Verification items for the finished model (mm, model axes). A direction names the side the tool comes from. Coordinates: 2 decimals unless noted, no trailing zeros. Write each loop counter-clockwise with the first axis right and the second up, starting at its lowest first coordinate (ties: lowest second). Pieces come first, ordered by that corner, then holes. Notation, with made-up numbers: (65, 59) -> (74, 59) arc R27 ccw to (74, 81) -> close; hole circle Ø7 at (27, -14). An arc over 180 degrees is marked (long way). Write item = value, one per line. Start each with the question number.
(1) Material ranges on probe 1 along X at (y, z) = (41, 1.5); probe 2 along Z at (x, y) = (8.4, 0), recorded low to high. Write a range as [from, to].
(2) Section check B-B (y = 0). Record the cut outline in (x, z).
(3) Set-up check for faces 1 (the face through (-8, -0.7, -5.4)), 2 (the face through (0, -1, -9.5)): record each of +Z, -Z, +X, -X, +Y, -Y from which the full face is reachable in a straight line by a thin tool's end or side.
(4) Section check C-C (x = -1.75). Record the cut outline in (y, z).
(5) Section check D-D (z = -3). Record the cut outline in (x, y), plus the area to 3 significant figures.
(6) Mould release check, pull along X, two halves, no side actions. Record for faces 3 (the face through (8, -0.7, -5.4)), 4 (the face through (9.5, -1, -6)), 5 (the face through (8.76, -1.08, -4.88)): released by +X, released by -X, zero draft, split by the parting line, or undercut.
(7) Gauge pin test, flat end, axial feed: pin 1 Ø3 at (x, z) = (3, -6) entering from -Y. Record the tip position at first contact, or that the pin passes through.
(8) Section check A-A (z = 6.5). Record the cut outline in (x, y), plus the area to 3 significant figures.
```python
from build123d import *

# Parameters (mm, degrees)
F0_W     = 19
F0_H     = 19
F0_W_2   = 16
F0_H_2   = 16
F2_DEPTH = 50
F1_R     = 5
F3_DEPTH = 12.5
F4_R     = 1


with BuildPart() as f2:
    # F0 (on Front) → F2 (new body, symmetric)
    with BuildSketch(Plane.XZ):
        Rectangle(F0_W, F0_H)
        Rectangle(F0_W_2, F0_H_2, mode=Mode.SUBTRACT)
    extrude(amount=F2_DEPTH, both=True)

    # F1 (on Right) → F3 (cut, symmetric)
    with BuildSketch(Plane.YZ):
        Circle(F1_R)
    extrude(amount=F3_DEPTH, both=True, mode=Mode.SUBTRACT)

    # F4
    f4_edges = [f2.edges().sort_by_distance(p)[0] for p in [
        (9.5, 0, 9.5),
        (-9.5, 0, 9.5),
        (9.5, 0, -9.5),
        (-9.5, 0, -9.5),
    ]]
    fillet(f4_edges, radius=F4_R)


solid = f2.part
```
Response:
q1.probe_1 = [-9.5, -8], [8, 9.5]
q1.probe_2 = [-9.5, -5], [5, 9.5]
q2.outline = (-9.5, -8.5) arc R1 ccw to (-8.5, -9.5) -> (8.5, -9.5) arc R1 ccw to (9.5, -8.5) -> (9.5, -5) -> (8, -5) -> (8, -8) -> (-8, -8) -> (-8, -5) -> (-9.5, -5) -> close; (-9.5, 5) -> (-8, 5) -> (-8, 8) -> (8, 8) -> (8, 5) -> (9.5, 5) -> (9.5, 8.5) arc R1 ccw to (8.5, 9.5) -> (-8.5, 9.5) arc R1 ccw to (-9.5, 8.5) -> close
q3.face_1 = +Y, -Y
q3.face_2 = -Z, +X, -X, +Y, -Y
q4.outline = (-50, -9.5) -> (50, -9.5) -> (50, -8) -> (-50, -8) -> close; (-50, 8) -> (50, 8) -> (50, 9.5) -> (-50, 9.5) -> close
q5.outline = (-9.5, -50) -> (-8, -50) -> (-8, -4) -> (-9.5, -4) -> close; (-9.5, 4) -> (-8, 4) -> (-8, 50) -> (-9.5, 50) -> close; (8, -50) -> (9.5, -50) -> (9.5, -4) -> (8, -4) -> close; (8, 4) -> (9.5, 4) -> (9.5, 50) -> (8, 50) -> close
q5.area = 276 mm2
q6.face_3 = undercut
q6.face_4 = released by +X
q6.face_5 = zero draft
q7.pin_1 = through
q8.outline = (-9.5, -50) -> (-8, -50) -> (-8, 50) -> (-9.5, 50) -> close; (8, -50) -> (9.5, -50) -> (9.5, 50) -> (8, 50) -> close
q8.area = 300 mm2
